Build history of the part. All positions in model axes, mm. A direction names the side the tool comes from. Give positions to 0.01 mm unless a question says otherwise; leave off trailing zeros. Write each loop counter-clockwise with the first axis right and the second up, starting at its lowest first coordinate (ties: lowest second). Pieces come first, ordered by that corner, then holes. Notation, with made-up numbers: (83.5, 5.5) -> (87.5, 5.5) arc R12 cw to (87.5, 9.5) -> close; hole circle Ø4 at (23.5, -5.75). An arc over 180 degrees is marked (long way). One line per question, with ' | ' between items. Start each with the question number.
(1) Band-saw the part on C-C, the plane x = 13. Give the cut face in (y, z).
(2) Band-saw the part on D-D, the plane y = 0. Give the cut face in (x, z).
(3) Pull direction X, two halves, no side cores. Call faces 1 (the flat face through (-1, -27.5, 1)), 2 (the flat face through (75, 0, 1)), 3 (the cylindrical face through (-71.32, -25.45, 1.48)): released by +X, released by -X, zero draft, split by the parting line, or undercut.
(4) Tool access for faces 4 (the cylindrical face through (46.93, 15.5, 7.44)), 5 (the flat face through (52, 15, 12)), 6 (the flat face through (-65, 0, 6)): list every direction of +Z, -Z, +X, -X, +Y, -Y with a clear straight run to the whole face (end or side of a thin tool).
(5) Pin check, flat tips, straight feed: P1, Ø4, axis at x = 0.5, z = 11, coming from the -Y side; P2, Ø3.5, axis at x = 72.75, y = -25, coming from the +Z side; P3, Ø8, axis at x = 52, y = 15, coming from the +Z side. Stop position of each tip, or through.
(6) Drill centre lines: probe 1 along Y at (x, z) = (72.75, 1.5); probe 2 along Z at (x, y) = (24.5, 8); probe 3 along Y at (x, z) = (-56.5, 5.5). Where is each one in solid material? Low to high. Write a range as from..to.
(7) Band-saw the part on B-B, the plane y = -7. Give the cut face in (x, z).
(8) Band-saw the part on A-A, the plane x = 72.75. Give the cut face in (y, z).
Solid Edge part; units mm, degrees
sketch "Sketch1" plane through (0, 0, 0) normal (0, 0, 1) x (1, 0, 0)
  circle A0 centre (-72.75, 25) radius 1.5
  circle A1 centre (72.75, 25) radius 1.5
  circle A2 centre (72.75, -25) radius 1.5
  circle A3 centre (-72.75, -25) radius 1.5
  line L0 (-75, -27.5) -> (75, -27.5)
  line L1 (75, -27.5) -> (75, 27.5)
  line L2 (75, 27.5) -> (-75, 27.5)
  line L3 (-75, 27.5) -> (-75, -27.5)
  dimension "D1" = 75
  dimension "D2" = 75
  dimension "D3" = 75
  dimension "D4" = 75
  dimension "D5" = 72.75
  dimension "D6" = 72.75
extrude "Protrusion1" add sketch "Sketch1" along normal blind 3
sketch "Sketch2" plane through (0, 0, 0) normal (0, 0, 1) x (1, 0, 0)
  line L0 (-65, -25) -> (30, -25)
  line L1 (30, -25) -> (30, 25)
  line L2 (30, 25) -> (-65, 25)
  line L3 (-65, 25) -> (-65, -25)
extrude "ExtrudedProtrusion_2" add sketch "Sketch2" along normal blind 10
sketch "Sketch3" plane through (0, 0, 0) normal (0, 0, 1) x (1, 0, 0)
  circle A0 centre (51.9265, 15.7222) radius 5
  circle A1 centre (51.9265, 15.7222) radius 0.5
extrude "ExtrudedProtrusion_3" add sketch "Sketch3" along normal blind 12
sketch "Sketch4" plane through (0, 0, 0) normal (0, 0, 1) x (1, 0, 0)
  line L0 (45, -5) -> (55, -5)
  line L1 (55, -5) -> (55, 5)
  line L2 (55, 5) -> (45, 5)
  line L3 (45, 5) -> (45, -5)
  dimension "D1" = 45
extrude "ExtrudedProtrusion_4" add sketch "Sketch4" along normal blind 7
sketch "Sketch5" plane through (50, 0, 7) normal (0, 0, 1) x (1, 0, 0)
  circle A0 centre (0, 0) radius 2.5
extrude "ExtrudedProtrusion_5" add sketch "Sketch5" along normal blind 11.1168
Results:
1) outline: (-27.5, 0) -> (27.5, 0) -> (27.5, 3) -> (25, 3) -> (25, 10) -> (-25, 10) -> (-25, 3) -> (-27.5, 3) -> close
2) outline: (-75, 0) -> (75, 0) -> (75, 3) -> (55, 3) -> (55, 7) -> (52.5, 7) -> (52.5, 18.12) -> (47.5, 18.12) -> (47.5, 7) -> (45, 7) -> (45, 3) -> (30, 3) -> (30, 10) -> (-65, 10) -> (-65, 3) -> (-75, 3) -> close
3) face 1: zero draft | face 2: released by +X | face 3: undercut
4) face 4: +Z | face 5: +Z, +X, -X, +Y | face 6: +Z, -X, +Y, -Y
5) P1: stops at y = -25 | P2: stops at z = 3 | P3: stops at z = 12
6) probe 1: y = -27.5..-26.5, -23.5..23.5, 26.5..27.5 | probe 2: z = 0..10 | probe 3: y = -25..25
7) outline: (-75, 0) -> (75, 0) -> (75, 3) -> (30, 3) -> (30, 10) -> (-65, 10) -> (-65, 3) -> (-75, 3) -> close
8) outline: (-27.5, 0) -> (-26.5, 0) -> (-26.5, 3) -> (-27.5, 3) -> close; (-23.5, 0) -> (23.5, 0) -> (23.5, 3) -> (-23.5, 3) -> close; (26.5, 0) -> (27.5, 0) -> (27.5, 3) -> (26.5, 3) -> close
